Input: part model. Units: mm. Frame: model coordinates. Face numbers are marked on the shaded views. A direction names the side the tool comes from. Give positions to 0.01 mm unless a question says otherwise; leave off trailing zeros. Loops run counter-clockwise (first coordinate to the right, second up) from the corner with the lowest first, then second, coordinate; pieces in that order, holes last. Notation, with made-up numbers: M 57.25,-32 L 81.25,-32 A28 ccw 81.25,-7 Z; hole C 4.5,23 d9. An arc over 180 degrees is marked long. Use a Markdown table: item, result. Add a question column.
from build123d import *

# Parameters (mm, degrees)
SKETCH_W     = 50
SKETCH_H     = 5
PAD_DEPTH    = 0.5
PAD001_DEPTH = 5


with BuildPart() as part:
    # Sketch → Pad (new body)
    with BuildSketch(Plane.XY):
        Rectangle(SKETCH_W, SKETCH_H)
    extrude(amount=PAD_DEPTH)

    # Sketch001 (on Face6 of Pad) → Pad001 (join)
    with BuildSketch(Plane.XY.offset(0.5)):
        with BuildLine():
            Line((-12.5, 1.1), (-22.5, 1.1))
            Line((-22.5, 1.1), (-22.5, -1.1))
            Line((-22.5, -1.1), (-12.5, -1.1))
            ThreePointArc((-12.5, -1.1), (-12.325514, -1.096955), (-12.151241, -1.087822))
            Line((-5.348759, -0.612178), (-12.151241, -1.087822))
            ThreePointArc((-5, -0.6), (-5.174486, -0.603045), (-5.348759, -0.612178))
            Line((5, -0.6), (-5, -0.6))
            ThreePointArc((5.348759, -0.612178), (5.174486, -0.603045), (5, -0.6))
            Line((5.348759, -0.612178), (12.151241, -1.087822))
            ThreePointArc((12.151241, -1.087822), (12.325514, -1.096955), (12.5, -1.1))
            Line((12.5, -1.1), (22.5, -1.1))
            Line((22.5, -1.1), (22.5, 1.1))
            Line((22.5, 1.1), (12.5, 1.1))
            ThreePointArc((12.5, 1.1), (12.325514, 1.096955), (12.151241, 1.087822))
            Line((5.348759, 0.612178), (12.151241, 1.087822))
            ThreePointArc((5, 0.6), (5.174486, 0.603045), (5.348759, 0.612178))
            Line((-5, 0.6), (5, 0.6))
            ThreePointArc((-5.348759, 0.612178), (-5.174486, 0.603045), (-5, 0.6))
            Line((-5.348759, 0.612178), (-12.151241, 1.087822))
            ThreePointArc((-12.151241, 1.087822), (-12.325514, 1.096955), (-12.5, 1.1))
        make_face()
    extrude(amount=PAD001_DEPTH)


solid = part.part
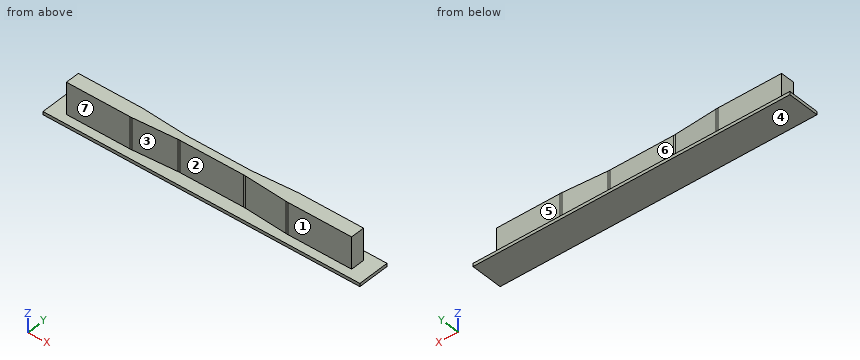
1) Section query B-B, the plane x = 3.5. Return the cut outline in (y, z), and give its area (3 significant figures).
2) Contact query for flat-ended pins moving along their axis: P1, Ø2, axis at x = -8, z = 5, coming from the -Y side; P2, Ø1.5, axis at x = -16.5, z = 3.5, coming from the -Y side; P3, Ø0.7, axis at y = 0.5, z = 3.5, coming from the -X side. Output: stop coordinate, or through.
3) Reachability of the marked faces 3, 4, 5, 6 and 7 from +Z, -Z, +X, -X, +Y, -Y: full face, straight path, thin tool, end or side. Return the list, or none.
4) Section query A-A, the plane y = 0.15. Return the cut outline in (x, z).
5) Pull-direction query (X, two-part tool) for the marked faces 1 and 2; classes: pulls with the +X half, pulls with the -X half, needs draft (parallel to the pull), parting line crosses it, or undercut.
6) Section query C-C, the plane z = 3.7. Return the cut outline in (x, y).
7) Ray query, line 1 (Y direction, x = -3, z = 3.6); line 2 (Y direction, x = -16.5, z = 1.15); line 3 (Z direction, x = -1, y = -0.95). Return the intervals inside material, ascending. Write a range as [from, to].
Entries:
| question | item | result |
|---|---|---|
| 1 | outline | M -2.5,0 L 2.5,0 L 2.5,0.5 L 0.6,0.5 L 0.6,5.5 L -0.6,5.5 L -0.6,0.5 L -2.5,0.5 Z |
| 1 | area | 8.50 mm² |
| 2 | P1 | stops at y = -0.87 |
| 2 | P2 | stops at y = -1.1 |
| 2 | P3 | stops at x = -22.5 |
| 3 | face 3 | +Z, -Y |
| 3 | face 4 | -Z, +X, -X, +Y, -Y |
| 3 | face 5 | +Z, +X, -X, +Y |
| 3 | face 6 | +Z, +Y |
| 3 | face 7 | +Z, +X, -X, -Y |
| 4 | outline | M -25,0 L 25,0 L 25,0.5 L 22.5,0.5 L 22.5,5.5 L -22.5,5.5 L -22.5,0.5 L -25,0.5 Z |
| 5 | face 1 | needs draft |
| 5 | face 2 | undercut |
| 6 | outline | M -22.5,-1.1 L -12.5,-1.1 A5 ccw -12.15,-1.09 L -5.35,-0.61 A5 cw -5,-0.6 L 5,-0.6 A5 cw 5.35,-0.61 L 12.15,-1.09 A5 ccw 12.5,-1.1 L 22.5,-1.1 L 22.5,1.1 L 12.5,1.1 A5 ccw 12.15,1.09 L 5.35,0.61 A5 cw 5,0.6 L -5,0.6 A5 cw -5.35,0.61 L -12.15,1.09 A5 ccw -12.5,1.1 L -22.5,1.1 Z |
| 7 | line 1 | y = [-0.6, 0.6] |
| 7 | line 2 | y = [-1.1, 1.1] |
| 7 | line 3 | z = [0, 0.5] |
